Read the model definition and answer for the solid it produces. Units are mm, in the model's axes. Face numbers are marked on the shaded views. A direction names the side the tool comes from. Coordinates: 2 decimals unless noted, no trailing zeros. Order: outer loops, then holes, each group sorted by start corner. A loop starts at its lowest first (then second) coordinate and runs counter-clockwise, first axis right, second up.
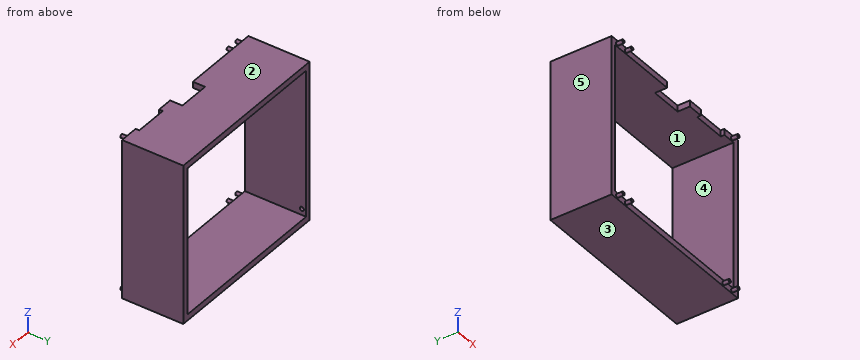
```python
from build123d import *

# Parameters (mm, degrees)
SKETCH1_W           = 72.25
SKETCH1_H           = 65
SKETCH1_W_2         = 67.75
SKETCH1_H_2         = 60
BOSS_EXTRUDE1_DEPTH = 25
SKETCH2_W           = 13
SKETCH2_H           = 5
SKETCH2_W_2         = 13.5
SKETCH2_H_2         = 1.5
CUT_EXTRUDE1_DEPTH  = 2.5
SKETCH5_R           = 0.7
BOSS_EXTRUDE2_DEPTH = 2.5
SKETCH7_R           = 0.85
CUT_EXTRUDE3_DEPTH  = 1.25
CUT_EXTRUDE4_START  = -1.25
SKETCH8_R           = 0.85
CUT_EXTRUDE4_DEPTH  = 1.25


with BuildPart() as part:
    # Sketch1 → Boss-Extrude1 (new body)
    with BuildSketch(Plane(origin=(0, 0, 0), x_dir=(1, 0, 0), z_dir=(0, 1, 0))):
        with Locations((36.125, -32.5)):
            Rectangle(SKETCH1_W, SKETCH1_H)
        with Locations((35.875, -32.5)):
            Rectangle(SKETCH1_W_2, SKETCH1_H_2, mode=Mode.SUBTRACT)
    extrude(amount=BOSS_EXTRUDE1_DEPTH)

    # Sketch2 → Cut-Extrude1 (cut)
    with BuildSketch(Plane.XY.offset(65)):
        with Locations((38.25, 2.5)):
            Rectangle(SKETCH2_W, SKETCH2_H)
        with Locations((57.75, 0.75)):
            Rectangle(SKETCH2_W_2, SKETCH2_H_2)
    extrude(amount=-CUT_EXTRUDE1_DEPTH, mode=Mode.SUBTRACT)

    # Sketch5 → Boss-Extrude2 (add)
    with BuildSketch(Plane.XZ):
        with Locations(Location((3.25, 63.722069184, 0), (0, 0, 90))):
            Circle(SKETCH5_R)
        with Locations(Location((8.25, 63.722069184, 0), (0, 0, 90))):
            Circle(SKETCH5_R)
        with Locations(Location((3.25, 1.277930816, 0), (0, 0, 90))):
            Circle(SKETCH5_R)
        with Locations(Location((8.25, 1.277930816, 0), (0, 0, 90))):
            Circle(SKETCH5_R)
        with Locations(Location((69, 63.722069184, 0), (0, 0, 90))):
            Circle(SKETCH5_R)
        with Locations(Location((69, 1.277930816, 0), (0, 0, 90))):
            Circle(SKETCH5_R)
        with Locations(Location((64, 1.277930816, 0), (0, 0, 90))):
            Circle(SKETCH5_R)
    extrude(amount=BOSS_EXTRUDE2_DEPTH)

    # Sketch7 → Cut-Extrude3 (cut)
    with BuildSketch(Plane.ZY.offset(-69.75)):
        with Locations((5, 23.25)):
            Circle(SKETCH7_R)
    extrude(amount=-CUT_EXTRUDE3_DEPTH, mode=Mode.SUBTRACT)

    # Sketch8 → Cut-Extrude4 (cut)
    with BuildSketch(Plane(origin=(2, 0, 0), x_dir=(0, 0, -1), z_dir=(1, 0, 0)).offset(CUT_EXTRUDE4_START)):
        with Locations(Location((-5, 23.25, 0), (0, 0, 180))):
            Circle(SKETCH8_R)
    extrude(amount=CUT_EXTRUDE4_DEPTH, mode=Mode.SUBTRACT)


solid = part.part
```
1) A cutting plane is placed at C-C, the plane x = 20. Determine the outline of the cut face in (y, z).
A:
outline: (0, 0) - (25, 0) - (25, 2.5) - (0, 2.5) - close; (0, 62.5) - (25, 62.5) - (25, 65) - (0, 65) - close
2) A cutting plane is placed at D-D, the plane z = 19. Determine the outline of the cut face in (x, y).
A:
outline: (0, 0) - (2, 0) - (2, 25) - (0, 25) - close; (69.75, 0) - (72.25, 0) - (72.25, 25) - (69.75, 25) - close
3) Flat-ended cylindrical pins translate along their axes: pin 1 Ø0.8 at (x, z) = (61, 63) entering from -Y; pin 2 Ø0.8 at (x, z) = (38, 64) entering from -Y; pin 3 Ø6 at (x, y) = (18.5, 5) entering from -Z; pin 4 Ø1.2 at (x, z) = (48.5, 63) entering from -Y. Find the tip coordinate at first contact, or state that the pin passes through.
A:
pin 1: stops at y = 1.5
pin 2: stops at y = 5
pin 3: stops at z = 0
pin 4: stops at y = 0
4) A cutting plane is placed at A-A, the plane z = 5. Determine the outline of the cut face in (x, y).
A:
outline: (0, 0) - (2, 0) - (2, 22.4) - (0.75, 22.4) - (0.75, 24.1) - (2, 24.1) - (2, 25) - (0, 25) - close; (69.75, 0) - (72.25, 0) - (72.25, 25) - (69.75, 25) - (69.75, 24.1) - (71, 24.1) - (71, 22.4) - (69.75, 22.4) - close
5) Which of the six approach directions +Z, -Z, +X, -X, +Y, -Y give full straight-line access (tool end or side, diameter ignored) to the marked faces 4 and 5?
A:
face 4: +Y, -Y
face 5: +Z, -Z, -X, +Y, -Y
6) A cutting plane is placed at B-B, the plane y = 23.25. Determine the outline of the cut face in (x, z).
A:
outline: (0, 0) - (72.25, 0) - (72.25, 65) - (0, 65) - close; hole (0.75, 4.15) - (2, 4.15) - (2, 2.5) - (69.75, 2.5) - (69.75, 4.15) - (71, 4.15) - (71, 5.85) - (69.75, 5.85) - (69.75, 62.5) - (2, 62.5) - (2, 5.85) - (0.75, 5.85) - close
7) Straight lines are drawn through the part: line 1 (Z direction, x = 47.5, y = 5.5); line 2 (X direction, y = 14.5, z = 52); line 3 (Y direction, x = 1.6, z = 5). For each, find the intervals that lie inside material, in ascending order.
A:
line 1: z = 0 to 2.5, 62.5 to 65
line 2: x = 0 to 2, 69.75 to 72.25
line 3: y = 0 to 22.4, 24.1 to 25
8) Determine the mould class of the marked faces 1, 2 and 3 for opening direction Z: pulls with the +Z half, pulls with the -Z half, needs draft (parallel to the pull), parting line crosses it, or undercut.
A:
face 1: undercut
face 2: pulls with the +Z half
face 3: pulls with the -Z half
